```python
from build123d import *

# Parameters (mm, degrees)
SKETCH2_R           = 19.05
SKETCH2_R_2         = 14.2875
SKETCH2_R_3         = 4.7625
SKETCH2_R_4         = 2.4892
BOSS_EXTRUDE1_DEPTH = 6.35
FILLET2_R           = 6.35


with BuildPart() as part:
    # Sketch2 → Boss-Extrude1 (new body)
    # profile 1 of 10: a face of its own
    with BuildSketch(Plane.XY):
        Circle(SKETCH2_R)
        Circle(SKETCH2_R_2, mode=Mode.SUBTRACT)
    # profile 2 of 10: a face of its own
    with BuildSketch(Plane.XY):
        with BuildLine():
            Line((30.461032527, -12.147828653), (18.828728894, -2.89507655))
            ThreePointArc((18.828728894, -2.89507655), (16.497783942, -9.525), (11.921574285, -14.858619268))
            Line((11.921574285, -14.858619268), (25.750844478, -20.306113668))
            ThreePointArc((25.750844478, -20.306113668), (23.371860585, -13.49375), (30.461032527, -12.147828653))
        make_face()
    # profile 3 of 10: a face of its own
    with BuildSketch(Plane.XY):
        with BuildLine():
            ThreePointArc((4.7625, 31.75), (-0.352941685, 27.000595993), (-4.710188049, 32.453942321))
            Line((-4.710188049, 32.453942321), (-6.907154609, 17.753695818))
            ThreePointArc((-6.907154609, 17.753695818), (0, 19.05), (6.907154609, 17.753695818))
            Line((6.907154609, 17.753695818), (4.710188049, 32.453942321))
            ThreePointArc((4.710188049, 32.453942321), (4.749404007, 32.102941685), (4.7625, 31.75))
        make_face()
    # profile 4 of 10: a face of its own
    with BuildSketch(Plane.XY):
        with BuildLine():
            ThreePointArc((-11.921574285, -14.858619268), (-16.497783942, -9.525), (-18.828728894, -2.89507655))
            Line((-18.828728894, -2.89507655), (-30.461032527, -12.147828653))
            ThreePointArc((-30.461032527, -12.147828653), (-25.427261032, -11.585424635), (-22.73380657, -15.875))
            ThreePointArc((-22.73380657, -15.875), (-23.55967289, -18.555358468), (-25.750844478, -20.306113668))
            Line((-25.750844478, -20.306113668), (-11.921574285, -14.858619268))
        make_face()
    # profile 5 of 10: a face of its own
    with BuildSketch(Plane.XY):
        with Locations((-27.49630657, -15.875)):
            Circle(SKETCH2_R_3)
        with Locations((-27.49630657, -15.875)):
            Circle(SKETCH2_R_4, mode=Mode.SUBTRACT)
    # profile 6 of 10: a face of its own
    with BuildSketch(Plane.XY):
        with Locations((27.49630657, -15.875)):
            Circle(SKETCH2_R_3)
        with Locations((27.49630657, -15.875)):
            Circle(SKETCH2_R_4, mode=Mode.SUBTRACT)
    # profile 7 of 10: a face of its own
    with BuildSketch(Plane.XY):
        with Locations((0, 31.75)):
            Circle(SKETCH2_R_3)
        with Locations((0, 31.75)):
            Circle(SKETCH2_R_4, mode=Mode.SUBTRACT)
    # profile 8 of 10: a face of its own
    with BuildSketch(Plane.XY):
        with BuildLine():
            ThreePointArc((6.907154609, 17.753695818), (0, 19.05), (-6.907154609, 17.753695818))
            ThreePointArc((-6.907154609, 17.753695818), (-16.497783942, 9.525), (-18.828728894, -2.89507655))
            ThreePointArc((-18.828728894, -2.89507655), (-16.497783942, -9.525), (-11.921574285, -14.858619268))
            ThreePointArc((-11.921574285, -14.858619268), (0, -19.05), (11.921574285, -14.858619268))
            ThreePointArc((11.921574285, -14.858619268), (16.497783942, -9.525), (18.828728894, -2.89507655))
            ThreePointArc((18.828728894, -2.89507655), (18.994601673, -1.451760064), (19.05, 0))
            ThreePointArc((19.05, 0), (15.723927552, 10.754561932), (6.907154609, 17.753695818))
        make_face()
        Circle(SKETCH2_R_2, mode=Mode.SUBTRACT)
    # profile 9 of 10: a face of its own
    with BuildSketch(Plane.XY):
        with BuildLine():
            ThreePointArc((6.907154609, 17.753695818), (0, 19.05), (-6.907154609, 17.753695818))
            ThreePointArc((-6.907154609, 17.753695818), (-16.497783942, 9.525), (-18.828728894, -2.89507655))
            ThreePointArc((-18.828728894, -2.89507655), (-16.497783942, -9.525), (-11.921574285, -14.858619268))
            ThreePointArc((-11.921574285, -14.858619268), (0, -19.05), (11.921574285, -14.858619268))
            ThreePointArc((11.921574285, -14.858619268), (16.497783942, -9.525), (18.828728894, -2.89507655))
            ThreePointArc((18.828728894, -2.89507655), (18.994601673, -1.451760064), (19.05, 0))
            ThreePointArc((19.05, 0), (15.723927552, 10.754561932), (6.907154609, 17.753695818))
        make_face()
        Circle(SKETCH2_R_2, mode=Mode.SUBTRACT)
    # profile 10 of 10: a face of its own
    with BuildSketch(Plane.XY):
        with BuildLine():
            ThreePointArc((6.907154609, 17.753695818), (0, 19.05), (-6.907154609, 17.753695818))
            ThreePointArc((-6.907154609, 17.753695818), (-16.497783942, 9.525), (-18.828728894, -2.89507655))
            ThreePointArc((-18.828728894, -2.89507655), (-16.497783942, -9.525), (-11.921574285, -14.858619268))
            ThreePointArc((-11.921574285, -14.858619268), (0, -19.05), (11.921574285, -14.858619268))
            ThreePointArc((11.921574285, -14.858619268), (16.497783942, -9.525), (18.828728894, -2.89507655))
            ThreePointArc((18.828728894, -2.89507655), (18.994601673, -1.451760064), (19.05, 0))
            ThreePointArc((19.05, 0), (15.723927552, 10.754561932), (6.907154609, 17.753695818))
        make_face()
        Circle(SKETCH2_R_2, mode=Mode.SUBTRACT)
    extrude(amount=BOSS_EXTRUDE1_DEPTH)

    # Fillet2
    fillet2_edges = [part.edges().sort_by_distance(p)[0] for p in [
        (18.828728894, -2.89507655, 3.175),
        (11.921574285, -14.858619268, 3.175),
        (-11.921574285, -14.858619268, 3.175),
        (-18.828728894, -2.89507655, 3.175),
        (-6.907154609, 17.753695818, 3.175),
        (6.907154609, 17.753695818, 3.175),
    ]]
    fillet(fillet2_edges, radius=FILLET2_R)


solid = part.part
```
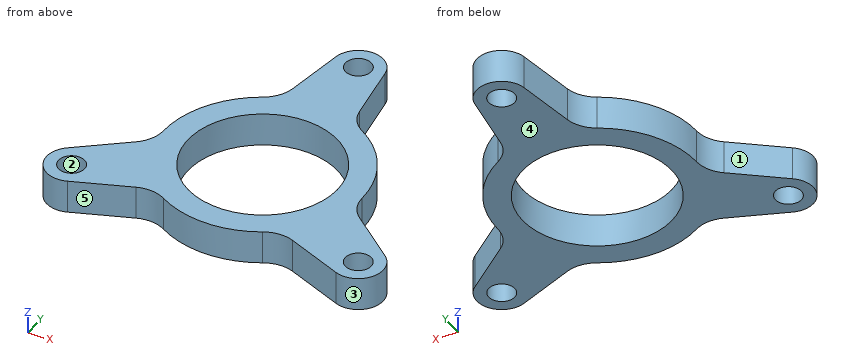
Model file for the job. Use its own axes, mm. Face numbers are marked on the shaded views. A direction names the side the tool comes from. Give positions to 0.01 mm unless a question says otherwise; leave off trailing zeros. Loops run counter-clockwise (first coordinate to the right, second up) from the corner with the lowest first, then second, coordinate; pieces in that order, holes last. Notation, with made-up numbers: (-27.5, 87.5) - (-0.5, 87.5) arc R31 ccw to (-0.5, 120.5) - close; hole circle Ø6 at (66, -22.75). An arc over 180 degrees is marked (long way). One line per item, written item: value. Start each with the question number.
1. Slice it at C-C (z = 1). Give the number of separate pieces and of enclosed holes in the cut face, plus the area to 3 significant figures.
2. Pull direction Y, two halves, no side cores. Call the marked faces 1, 2 and 3: pulls with the +Y half, pulls with the -Y half, needs draft (parallel to the pull), parting line crosses it, or undercut.
3. Pin check, flat tips, straight feed: pin 1 (3 mm diameter, centred on y = -13.5, z = 4.5, fed in from -X); pin 2 (2 mm diameter, centred on x = 14.5, z = 1.5, fed in from -Y). Stop position of each tip, or through.
4. Slice it at B-B (y = 4). List the corners of the cut face in (x, z), plus the area to 3 significant figures.
5. Slice it at D-D (y = 26.5). List the corners of the cut face in (x, z), plus the area to 3 significant figures.
6. Which spindle directions (+Z, -Z, +X, -X, +Y, -Y) get a long thin tool onto all of the face, cutting with end or side? Do the marked faces 4 and 5. Say none if no direction does.
7. Probe L1, parallel to Y at x = 0, z = 2.25; L2, parallel to X at y = -8.5, z = 4.5; L3, parallel to Y at x = 27, z = 0.5. List the from-to ranges inside material, lowest first. Write a range as from..to.
8. Slice it at A-A (x = 0). List the corners of the cut face in (y, z), plus the area to 3 significant figures.
Solution:
1. separate pieces: 1
1. enclosed holes: 4
1. area: 1,010 mm^2
2. face 1: pulls with the +Y half
2. face 2: undercut
2. face 3: parting line crosses it
3. pin 1: stops at x = -32.18
3. pin 2: stops at y = -16.27
4. outline: (-18.63, 0) - (-13.72, 0) - (-13.72, 6.35) - (-18.63, 6.35) - close; (13.72, 0) - (18.63, 0) - (18.63, 6.35) - (13.72, 6.35) - close
4. area: 62.3 mm^2
5. outline: (-5.6, 0) - (5.6, 0) - (5.6, 6.35) - (-5.6, 6.35) - close
5. area: 71.1 mm^2
6. face 4: -Z, +X, -X, +Y, -Y
6. face 5: +Z, -Z, -Y
7. L1: y = -19.05..-14.29, 14.29..29.26, 34.24..36.51
7. L2: x = -25.88..-11.48, 11.48..25.88
7. L3: y = -20.61..-18.31, -13.44..-9.39
8. outline: (-19.05, 0) - (-14.29, 0) - (-14.29, 6.35) - (-19.05, 6.35) - close; (14.29, 0) - (29.26, 0) - (29.26, 6.35) - (14.29, 6.35) - close; (34.24, 0) - (36.51, 0) - (36.51, 6.35) - (34.24, 6.35) - close
8. area: 140 mm^2
